from build123d import *

# Parameters (mm, degrees)
SKETCH_1_R          = 8
EXTRUDE_1_DEPTH     = 8
SKETCH_2_R          = 6
CUT_EXTRUDE_1_DEPTH = 6
SKETCH_3_R          = 1.5
CUT_EXTRUDE_2_DEPTH = 14.856406461


with BuildPart() as part:
    # 草图1 → 凸台-拉伸1 (new body)
    with BuildSketch(Plane.XY):
        Circle(SKETCH_1_R)
    extrude(amount=EXTRUDE_1_DEPTH)

    # 草图2 → 切除-拉伸1 (cut)
    with BuildSketch(Plane(origin=(0, 0, 0), x_dir=(-1, 0, 0), z_dir=(0, 0, -1))):
        Circle(SKETCH_2_R)
    extrude(amount=-CUT_EXTRUDE_1_DEPTH, mode=Mode.SUBTRACT)

    # 草图3 → 切除-拉伸2 (cut, through all)
    with BuildSketch(Plane.XY.offset(8)):
        Circle(SKETCH_3_R)
    extrude(amount=-CUT_EXTRUDE_2_DEPTH, mode=Mode.SUBTRACT)


solid = part.part
Build history of the part. All positions in model axes, mm. A direction names the side the tool comes from. Coordinates: 2 decimals unless noted, no trailing zeros. Write each loop counter-clockwise with the first axis right and the second up, starting at its lowest first coordinate (ties: lowest second). Pieces come first, ordered by that corner, then holes.
(1) 3-axis set-ups, long thin cutter, end or side, ignore diameter. For faces 4 (the cylindrical face through (6, 0, 3)), 5 (the flat face through (2, 0, 8)): which of +Z, -Z, +X, -X, +Y, -Y reach the whole face in a straight line?
(2) Drill centre lines: line 1 (Y direction, x = 0, z = 7.4); line 2 (Y direction, x = 0, z = 1.95); line 3 (Z direction, x = -3.5, y = 2.5). Where is each one in solid material? Low to high.
(3) Cut at A-A on x = 0. List the corners of the cut face in (y, z), and give its area (3 significant figures).
(4) Cut at D-D on x = 3. List the corners of the cut face in (y, z).
(5) Mould opens along Y. For faces 1 (the cylindrical face through (-1.5, 0.07, 7.01)), 2 (the cylindrical face through (-1.73, -7.81, 3.94)), 3 (the flat face through (-2, 6, 0)) say: pulls with the +Y half, pulls with the -Y half, needs draft (parallel to the pull), parting line crosses it, or undercut.
(6) Cut at C-C on z = 3. List the corners of the cut face in (x, y).
(7) Pin check, flat tips, straight feed: pin 1 Ø1 at (x, z) = (-5.5, 1.5) entering from +Y (3 decimals); pin 2 Ø3.5 at (x, y) = (-0.5, -1.5) entering from -Z; pin 3 Ø3 at (y, z) = (3.5, 3) entering from -X. Stop position of each tip, or through.
Working result:
1. face 4: -Z
1. face 5: +Z, +X, -X, +Y, -Y
2. line 1: y = -8 to -1.5, 1.5 to 8
2. line 2: y = -8 to -6, 6 to 8
2. line 3: z = 6 to 8
3. outline: (-8, 0) - (-6, 0) - (-6, 6) - (-1.5, 6) - (-1.5, 8) - (-8, 8) - close; (1.5, 6) - (6, 6) - (6, 0) - (8, 0) - (8, 8) - (1.5, 8) - close
3. area: 50.0 mm2
4. outline: (-7.42, 0) - (-5.2, 0) - (-5.2, 6) - (5.2, 6) - (5.2, 0) - (7.42, 0) - (7.42, 8) - (-7.42, 8) - close
5. face 1: undercut
5. face 2: parting line crosses it
5. face 3: needs draft
6. outline: circle Ø16 at (0, 0); hole circle Ø12 at (0, 0)
7. pin 1: stops at y = 6.245
7. pin 2: stops at z = 6
7. pin 3: stops at x = -7.75
